from build123d import *

# Parameters (mm, degrees)
F1_DEPTH = 12.7
F2_T     = -5.08


with BuildPart() as f1:
    # F0 (on Top) → F1 (new body)
    with BuildSketch(Plane.XY):
        Polygon((-127.572568, 155.790623), (-79.69885, -15.442981), (110.80115, -15.442981), (151.827432, 157.558996), align=None)
    extrude(amount=F1_DEPTH)

    # F2
    f2_openings = [f1.faces().sort_by_distance(p)[0] for p in [
        (13.894392, 76.045407, 12.7),
    ]]
    offset(amount=F2_T, openings=f2_openings)


solid = f1.part
Check sheet for the modelled part. Datum: model origin and axes. Units: mm. A direction names the side the tool comes from. Round coordinates to 2 decimals unless told otherwise and drop trailing zeros. Order: outer loops, then holes, each group sorted by start corner. A loop starts at its lowest first (then second) coordinate and runs counter-clockwise, first axis right, second up.
(1) Cross-section at A-A, the plane z = 8.25. Enter the section's corners in (x, y), and give its area (3 significant figures).
(2) Go/stop test with flat-tipped pins: P1, Ø2, axis at x = -37, z = 10, coming from the +Y side; P2, Ø6, axis at y = 129.5, z = 7.5, coming from the +X side; P3, Ø6, axis at y = 12, z = 3.5, coming from the +X side. Record where each tip stops, or that it passes through.
(3) Access from +Z, -Z, +X, -X, +Y, -Y to the whole of each face (thin tool, end or side, straight path). Record for faces 1 (the flat face through (131.027, 69.847, 6.261)), 2 (the flat face through (125.82, 69.9, 8.84)).
(4) Cross-section at C-C, the plane y = 110. Enter the section's corners in (x, z), and give its area (3 significant figures).
(5) Cross-section at B-B, the plane x = 38. Enter the section's corners in (y, z).
(6) Draft check along Y on faces 3 (the flat face through (10, 72, 0)), 4 (the flat face through (14, -10.363, 9)), 5 (the flat face through (-103.97, 71.37, 6.26)). Enter one of: pulls with the +Y half, pulls with the -Y half, needs draft (parallel to the pull), parting line crosses it, or undercut.
(7) Scan lines: probe 1 along X at (y, z) = (12, 7.75); probe 2 along Z at (x, y) = (117.5, 71.5); probe 3 along X at (y, z) = (54, 9.75). Record each from-to range of solid material in increasing order.
Check sheet entries:
1. outline: (-127.57, 155.79) - (-79.7, -15.44) - (110.8, -15.44) - (151.83, 157.56) - close; hole (-120.89, 150.75) - (-75.84, -10.36) - (106.78, -10.36) - (145.39, 152.44) - close
1. area: 4,090 mm2
2. P1: stops at y = 156.37
2. P2: stops at x = 145.88
2. P3: stops at x = 118.02
3. face 1: +Z, -Z, +X, -Y
3. face 2: +Z
4. outline: (-114.77, 0) - (140.55, 0) - (140.55, 12.7) - (135.33, 12.7) - (135.33, 5.08) - (-109.5, 5.08) - (-109.5, 12.7) - (-114.77, 12.7) - close
4. area: 1,380 mm2
5. outline: (-15.44, 0) - (156.84, 0) - (156.84, 12.7) - (151.76, 12.7) - (151.76, 5.08) - (-10.36, 5.08) - (-10.36, 12.7) - (-15.44, 12.7) - close
6. face 3: needs draft
6. face 4: undercut
6. face 5: pulls with the -Y half
7. probe 1: x = -87.37 to -82.1, 112.09 to 117.31
7. probe 2: z = 0 to 5.08
7. probe 3: x = -99.11 to -93.84, 122.05 to 127.27
